Geometry: final body of the model. Coordinates: model frame, mm. Round coordinates to 2 decimals unless told otherwise and drop trailing zeros. Loops run counter-clockwise (first coordinate to the right, second up) from the corner with the lowest first, then second, coordinate; pieces in that order, holes last. Notation, with made-up numbers: (42, 60) - (82, 60) arc R22 cw to (82, 89) - close; hole circle Ø4 at (18, -14.5). An arc over 180 degrees is marked (long way). Return JSON: item names as keys, results as strings. Group by question number.
1. Material intervals for probe 1 along Y at (x, z) = (2.65, -134); probe 2 along Y at (x, z) = (1.35, -107.95); probe 3 along Z at (x, y) = (0.3, 14), sorted ascending.
2. Section C-C on x = 0.95. Return loops of the section in (y, z) (3 decimals).
3. Section D-D on z = -69. Return loops of the section in (x, y) (3 decimals).
4. Section A-A on y = 12.7. Return loops of the section in (x, z) (3 decimals).
5. First-contact query: pin 1 Ø8 at (y, z) = (225.42, -116.55) entering from -X; pin 2 Ø6 at (y, z) = (12.7, -107.95) entering from +X. Flat tips, straight axial feed; report the tip coordinate or a pass-through.
6. Section B-B on z = -12.7. Return loops of the section in (x, y) (3 decimals).
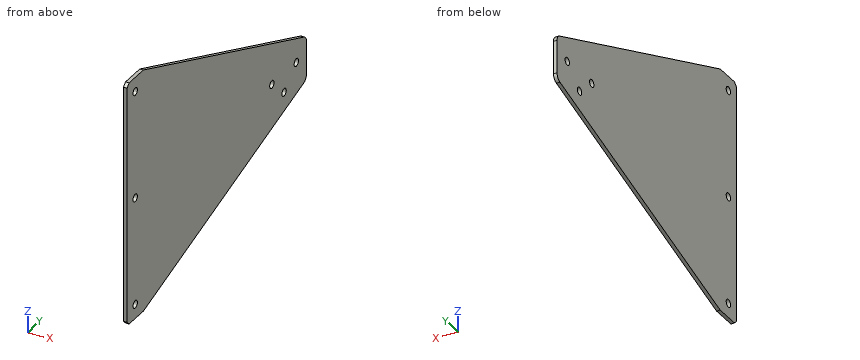
from build123d import *

# Parameters (mm, degrees)
BOSS_EXTRUDE1_DEPTH = 3.175
SKETCH3_R           = 3.3782
CUT_EXTRUDE2_DEPTH  = 354.110819184
SKETCH4_R           = 3.3782
CUT_EXTRUDE3_DEPTH  = 354.110819184
CHAMFER1_SIZE       = 3.175


with BuildPart() as part:
    # Sketch1 → Boss-Extrude1 (new body)
    with BuildSketch(Plane(origin=(0, 0, 0), x_dir=(0, 0, -1), z_dir=(1, 0, 0))):
        with BuildLine():
            Line((105.899159305, 279.4), (134.975405367, 279.4))
            ThreePointArc((134.975405367, 279.4), (138.76591423, 278.144560095), (141.057602278, 274.874659073))
            Line((141.057602278, 274.874659073), (215.9, 25.4))
            Line((215.9, 25.4), (215.9, 0))
            Line((215.9, 0), (0, 0))
            Line((0, 0), (0, 25.4))
            Line((0, 25.4), (100.003332318, 275.408330795))
            ThreePointArc((100.003332318, 275.408330795), (102.339166366, 278.308226913), (105.899159305, 279.4))
        make_face()
    extrude(amount=BOSS_EXTRUDE1_DEPTH)

    # Sketch3 → Cut-Extrude2 (cut, through all)
    with BuildSketch(Plane(origin=(3.175, 0, 0), x_dir=(0, 0, -1), z_dir=(1, 0, 0))):
        with Locations((133.35, 244.475)):
            Circle(SKETCH3_R)
        with Locations((116.549479175, 225.425)):
            Circle(SKETCH3_R)
        with Locations((116.549479175, 263.525)):
            Circle(SKETCH3_R)
    extrude(amount=-CUT_EXTRUDE2_DEPTH, mode=Mode.SUBTRACT)

    # Sketch4 → Cut-Extrude3 (cut, through all)
    with BuildSketch(Plane(origin=(3.175, 0, 0), x_dir=(0, 0, -1), z_dir=(1, 0, 0))):
        with Locations((12.7, 12.7)):
            Circle(SKETCH4_R)
        with Locations((107.95, 12.7)):
            Circle(SKETCH4_R)
        with Locations((203.2, 12.7)):
            Circle(SKETCH4_R)
    extrude(amount=-CUT_EXTRUDE3_DEPTH, mode=Mode.SUBTRACT)

    # Chamfer1
    chamfer1_edges = [part.edges().sort_by_distance(p)[0] for p in [
        (1.5875, 0, -215.9),
        (1.5875, 0, 0),
    ]]
    chamfer(chamfer1_edges, length=CHAMFER1_SIZE)


solid = part.part
Taken from the geometry:
{
 "1": {"probe 1": "0 to 241.16, 247.79 to 279.4", "probe 2": "0 to 9.32, 16.08 to 279.4", "probe 3": "-215.9 to -206.32, -200.08 to -111.07, -104.83 to -15.82, -9.58 to 0"},
 "2": {"outline": "(0, -212.725) - (3.175, -215.9) - (25.4, -215.9) - (274.875, -141.058) arc R6.35 ccw to (279.4, -134.975) - (279.4, -105.899) arc R6.35 ccw to (275.408, -100.003) - (25.4, 0) - (3.175, 0) - (0, -3.175) - close; hole circle Ø6.756 at (12.7, -203.2); hole circle Ø6.756 at (12.7, -107.95); hole circle Ø6.756 at (12.7, -12.7); hole circle Ø6.756 at (225.425, -116.549); hole circle Ø6.756 at (244.475, -133.35); hole circle Ø6.756 at (263.525, -116.549)"},
 "3": {"outline": "(0, 0) - (3.175, 0) - (3.175, 197.9) - (0, 197.9) - close"},
 "4": {"outline": "(0, -215.9) - (3.175, -215.9) - (3.175, -206.578) - (0, -206.578) - close; (0, -199.822) - (3.175, -199.822) - (3.175, -111.328) - (0, -111.328) - close; (0, -104.572) - (3.175, -104.572) - (3.175, -16.078) - (0, -16.078) - close; (0, -9.322) - (3.175, -9.322) - (3.175, 0) - (0, 0) - close"},
 "5": {"pin 1": "x = 0", "pin 2": "through"},
 "6": {"outline": "(0, 0) - (3.175, 0) - (3.175, 9.322) - (0, 9.322) - close; (0, 16.078) - (3.175, 16.078) - (3.175, 57.15) - (0, 57.15) - close"}
}
